Could you check a few things on this drawing? It's one solid part, dimensions in mm from its lowest x, y, z. A direction names the side the tool comes from. Coordinates: 2 decimals unless noted, no trailing zeros. Write each loop counter-clockwise with the first axis right and the second up, starting at its lowest first coordinate (ties: lowest second). Pieces come first, ordered by that corner, then holes. Notation, with made-up numbers: (23.5, -17.5) - (60.5, -17.5) arc R20 ccw to (60.5, 4.5) - close; hole circle Ø10 at (11.25, 12.25). An arc over 180 degrees is marked (long way). Use one line per item in the form item = value. Start each with the question number.
(1) On a 3-axis mill with a long thin cutter (end or side, diameter ignored), from which of +Z, -Z, +X, -X, +Y, -Y can I reach the whole of each face in a straight line? I mean the marked faces 1 and 2. Say none if no direction works.
(2) If we section it at C-C on y = 40: Please give me the cut outline in (x, z).
(3) If we section it at A-A on x = 6: Please give me the cut outline in (y, z) (1 decimal), then the cut area to 3 significant figures.
(4) If we section it at D-D on x = 20.5: Please give me the cut outline in (y, z), then the cut area to 3 significant figures.
(5) For pin 1 Ø10 at (x, z) = (26, 24.5) entering from -Y; pin 2 Ø2.5 at (y, z) = (50.5, 10.5) entering from -X; pin 3 Ø5 at (x, y) = (4, 12) entering from +Z; pin 4 Ø1.5 at (y, z) = (21, 4) entering from -X, each with a flat end and sliding along its axis, tell me the tip position at first contact or that it passes through.
(6) If we section it at B-B on z = 11: Please give me the cut outline in (x, y), then the cut area to 3 significant figures.
(7) If I drill on probe 1 along X at (y, z) = (50, 11.5); probe 2 along Z at (x, y) = (23, 8.5); probe 3 along Y at (x, z) = (20, 20.5), over which ranges is the centre line in solid material (lowest first)? Write a range as from..to.
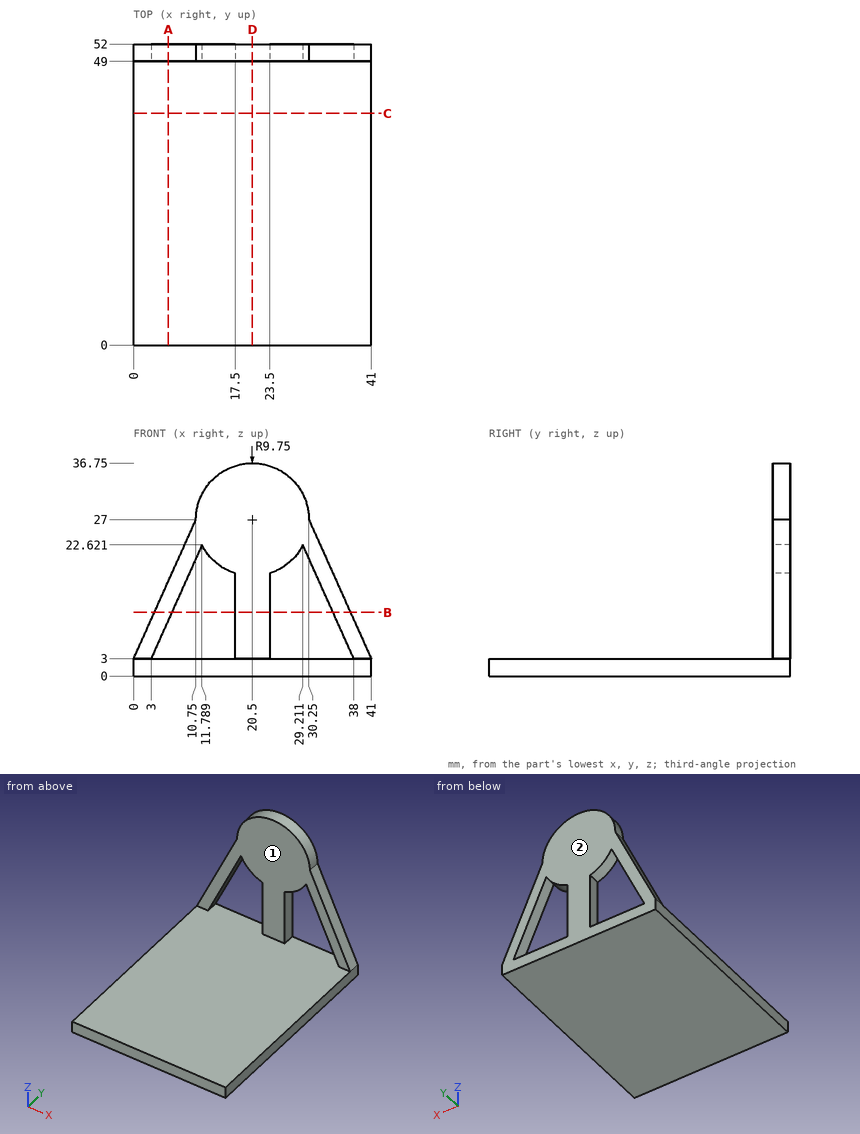
Reported:
q1.face_1 = +Z, +X, -X, -Y
q1.face_2 = +Z, -Z, +X, -X, +Y
q2.outline = (0, 0) - (41, 0) - (41, 3) - (0, 3) - close
q3.outline = (0, 0) - (52, 0) - (52, 3) - (0, 3) - close; (49, 9.7) - (52, 9.7) - (52, 16.4) - (49, 16.4) - close
q3.area = 176 mm2
q4.outline = (0, 0) - (52, 0) - (52, 36.75) - (49, 36.75) - (49, 3) - (0, 3) - close
q4.area = 257 mm2
q5.pin_1 = 49
q5.pin_2 = 2.8
q5.pin_3 = 3
q5.pin_4 = through
q6.outline = (3.58, 49) - (6.58, 49) - (6.58, 52) - (3.58, 52) - close; (17.5, 49) - (23.5, 49) - (23.5, 52) - (17.5, 52) - close; (34.42, 49) - (37.42, 49) - (37.42, 52) - (34.42, 52) - close
q6.area = 36.0 mm2
q7.probe_1 = 3.81..6.81, 17.5..23.5, 34.19..37.19
q7.probe_2 = 0..3
q7.probe_3 = 49..52
